Drawing for the job (mm, zero at the part's lowest x, y, z). Coordinates: 2 decimals unless noted, no trailing zeros. Write each loop counter-clockwise with the first axis right and the second up, starting at its lowest first coordinate (ties: lowest second). Pieces come first, ordered by that corner, then holes. Notation, with made-up numbers: M -8.5,72 L 27.5,72 A17 cw 27.5,100 Z; hole C 79.25,28 d9. An arc over 180 degrees is marked long. Put each result on its own line as item: value. Start each with the question number.
Q1. Drop flat-ended pins along their axis: pin 1 (6.5 mm diameter, centred on y = 23, z = 7, fed in from -X); pin 2 (4 mm diameter, centred on x = 20.5, z = 4.5, fed in from +Y). Give the stop position or say it passes through.
Q2. Cut at B-B (y = 438). Write the cut outline in (x, z), then the cut area to 3 significant figures.
Q3. Cut at C-C (x = 196.5). Write the cut outline in (y, z), then the cut area to 3 significant figures.
Q4. Cut at D-D (z = 7). Give the number of separate pieces and of enclosed holes in the cut face, then the cut area to 3 significant figures.
Q5. Drill centre lines: line 1 along Y through (x, z) = (208.5, 6); line 2 along Y through (x, z) = (116.5, 11); line 3 along X through (y, z) = (431.5, 10.25). Where is each one in solid material? Low to high.
Q6. Cut at A-A (x = 108.5). Write the cut outline in (y, z), then the cut area to 3 significant figures.
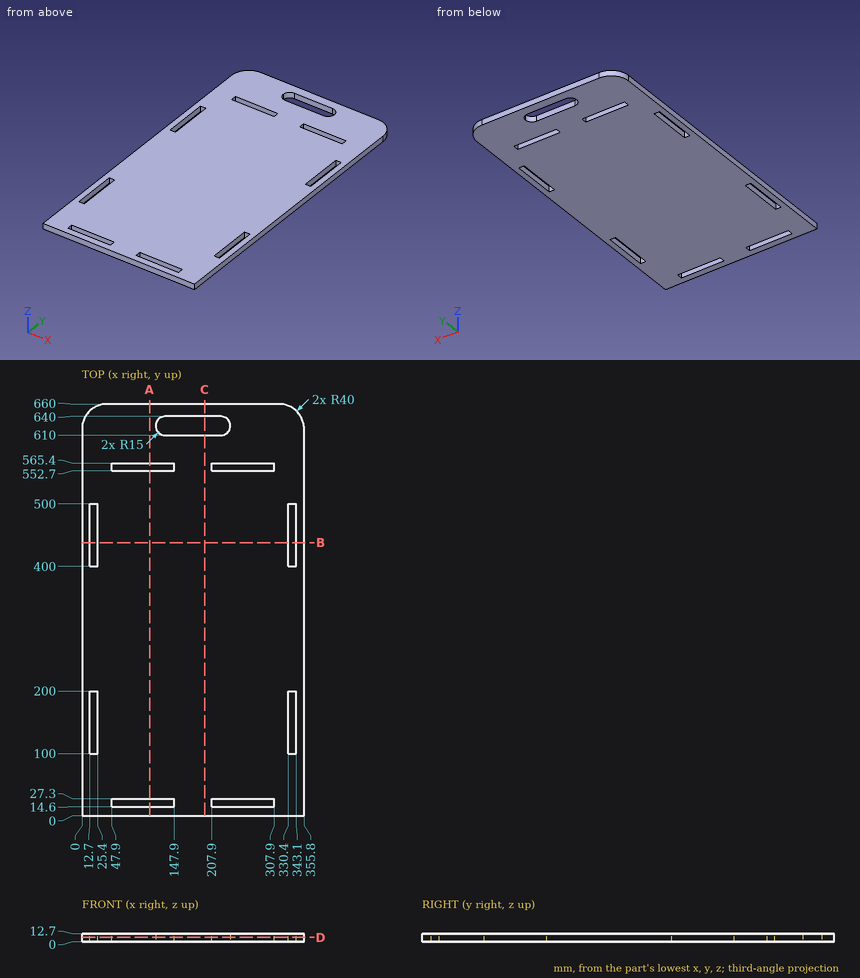
Computed values:
1. pin 1: x = 0
1. pin 2: y = 655.97
2. outline: M 0,0 L 12.7,0 L 12.7,12.7 L 0,12.7 Z; M 25.4,0 L 330.4,0 L 330.4,12.7 L 25.4,12.7 Z; M 343.1,0 L 355.8,0 L 355.8,12.7 L 343.1,12.7 Z
2. area: 4,200 mm2
3. outline: M 0,0 L 610,0 L 610,12.7 L 0,12.7 Z; M 640,0 L 660,0 L 660,12.7 L 640,12.7 Z
3. area: 8,000 mm2
4. separate pieces: 1
4. enclosed holes: 9
4. area: 221,000 mm2
5. line 1: 0 to 14.6, 27.3 to 552.7, 565.4 to 610, 640 to 660
5. line 2: 0 to 14.6, 27.3 to 552.7, 565.4 to 660
5. line 3: 0 to 12.7, 25.4 to 330.4, 343.1 to 355.8
6. outline: M 0,0 L 14.6,0 L 14.6,12.7 L 0,12.7 Z; M 27.3,0 L 552.7,0 L 552.7,12.7 L 27.3,12.7 Z; M 565.4,0 L 660,0 L 660,12.7 L 565.4,12.7 Z
6. area: 8,060 mm2
